The listing builds one solid part. Answer for the finished solid, in the listing's coordinates (mm). Round coordinates to 2 decimals unless told otherwise and drop trailing zeros. Write each loop counter-clockwise with the first axis right and the second up, starting at its lowest first coordinate (ties: lowest second). Pieces come first, ordered by that corner, then holes. Notation, with made-up numbers: M -26,-22 L -15,-22 A30 cw -15,16 Z; hole C -6.5,-30.75 d10. An arc over 180 degrees is marked long. Write each question's results on one line, items separated by ' | '.
Autodesk Inventor part; units mm, degrees
ref_plane "YZ Plane" through (0, 0, 0) normal (1, 0, 0) x (0, 1, 0)
ref_plane "XZ Plane" through (0, 0, 0) normal (0, 1, 0) x (-1, 0, 0)
ref_plane "XY Plane" through (0, 0, 0) normal (0, 0, 1) x (1, 0, 0)
sketch "スケッチ1" plane through (0, 0, 0) normal (0, 1, 0) x (-1, 0, 0)
  circle A0 centre (0, 0) radius 86.2565
  circle A1 centre (0, 0) radius 7.5
  dimension "d0" = 172.513
  dimension "d1" = 15
extrude "押し出し1" add sketch "スケッチ1" along normal blind 3
sketch "スケッチ2" plane through (0, 3, 0) normal (0, 1, 0) x (1, 0, 0)
  circle A0 centre (0, 0) radius 50.75
  point P0 (0, 50.75)
  point P1 (-50.75, 0)
  point P2 (0, -50.75)
  point P3 (50.75, 0)
  dimension "d4" = 101.5
  dimension "d7" = 360
hole "穴1" at (0, 3, -50.75) at (-50.75, 3, 0) at (0, 3, 50.75) at (50.75, 3, 0) direction (0, -1, 0) diameter 4.3 end through all
sketch "スケッチ3" plane through (0, 3, 0) normal (0, 1, 0) x (1, 0, 0)
  line L0 (0, 0) -> (86.2565, 0)
  circle A0 centre (0, 0) radius 86.2565
  circle A1 centre (0, 0) radius 7.5
  line L1 (0, 0) -> (60.9926, -60.9926)
  line L2 (-8.1772, -85.868) -> (-85.868, -8.1772)
  line L3 (85.868, 8.1772) -> (8.1772, 85.868)
  point P0 (8.1772, 85.868)
  point P1 (83.085, 0)
  point P2 (85.868, 8.1772)
  dimension "d16" = 45
  dimension "d64" = 66.5
extrude "押し出し2" cut sketch "スケッチ3" against normal blind 3 contours L3 A0 | A0 L2
sketch "スケッチ4" plane through (0, 3, 0) normal (0, 1, 0) x (1, 0, 0)
  circle A0 centre (0, 0) radius 7.5
  circle A1 centre (0, 0) radius 12
  line L0 (0, 0) -> (-8.4853, -8.4853)
  line L1 (0, 0) -> (-12, 0)
  point P0 (3.1058, -11.5911)
  point P1 (11.5911, -3.1058)
  point P2 (8.4853, 8.4853)
  point P3 (-3.1058, 11.5911)
  point P4 (-11.5911, 3.1058)
  dimension "d20" = 24
  dimension "d21" = 45
  dimension "d24" = 360
hole "穴2" at (-8.4853, 3, 8.4853) at (3.1058, 3, 11.5911) at (11.5911, 3, 3.1058) at (8.4853, 3, -8.4853) at (-3.1058, 3, -11.5911) at (-11.5911, 3, -3.1058) direction (0, -1, 0) diameter 4.3 end through all
sketch "スケッチ5" plane through (0, 3, 0) normal (0, 1, 0) x (1, 0, 0)
  arc A0 (-8.1772, -85.868) -> (85.868, 8.1772) centre (0, 0) ccw
  line L0 (5.2626, -86.0958) -> (-86.0958, 5.2626)
  arc A1 (8.1772, 85.868) -> (-85.868, -8.1772) centre (0, 0) ccw
  line L1 (-85.868, -8.1772) -> (-8.1772, -85.868)
  line L2 (-5.2626, 86.0958) -> (86.0958, -5.2626)
  line L3 (85.868, 8.1772) -> (8.1772, 85.868)
  line L4 (-85.868, -8.1772) -> (8.1772, 85.868)
  line L5 (-8.1772, -85.868) -> (85.868, 8.1772)
  line L6 (-73.6506, -7.1826) -> (7.1826, 73.6506)
  line L7 (80.2566, 13.7886) -> (-7.1826, -73.6506)
  line L8 (0, 0) -> (40.4166, 40.4166)
  circle A2 centre (0, 0) radius 74
  point P0 (-73.6506, -7.1826)
  point P1 (7.1826, 73.6506)
  point P2 (73.6506, 7.1826)
  dimension "d61" = 148
  dimension "d62" = 47
  dimension "d63" = 47
hole "穴3" at (-73.6506, 3, 7.1826) at (7.1826, 3, -73.6506) at (73.6506, 3, -7.1826) at (-7.1826, 3, 73.6506) direction (0, -1, 0) diameter 3.2 end through all
sketch "スケッチ6" plane through (0, 3, 0) normal (0, 1, 0) x (1, 0, 0)
  circle A0 centre (0, 0) radius 7.5
  circle A1 centre (0, 0) radius 70
  circle A2 centre (0, 0) radius 50
  circle A3 centre (7.1826, 73.6506) radius 1.6
  line L0 (0, 0) -> (7.1826, 73.6506)
  circle A4 centre (-73.6506, -7.1826) radius 1.6
  line L1 (0, 0) -> (-73.6506, -7.1826)
  line L2 (0, 0) -> (-11.469, 69.0541)
  line L3 (0, 0) -> (-69.0541, 11.469)
  circle A5 centre (0, 0) radius 25
  circle A6 centre (0, 50.75) radius 2.15
  line L4 (0, 0) -> (0, 50.75)
  line L5 (0, 0) -> (8.6824, 49.2404)
  line L6 (0, 0) -> (49.2404, 8.6824)
  circle A7 centre (50.75, 0) radius 2.15
  line L7 (0, 0) -> (50.75, 0)
  line L8 (0, 0) -> (-49.2404, -8.6824)
  line L9 (0, 0) -> (-8.6824, -49.2404)
  line L10 (0, 0) -> (11.469, -69.0541)
  line L11 (0, 0) -> (69.0541, -11.469)
  circle A8 centre (0, 0) radius 40
  point P0 (-4.3412, -24.6202)
  point P1 (-24.6202, -4.3412)
  point P2 (49.3243, -8.1921)
  point P3 (24.6622, -4.0961)
  point P4 (4.0961, -24.6622)
  point P5 (8.1921, -49.3243)
  point P6 (24.6202, 4.3412)
  point P7 (4.3412, 24.6202)
  point P8 (-24.6622, 4.0961)
  point P9 (-4.0961, 24.6622)
  point P10 (-8.1921, 49.3243)
  point P11 (-49.3243, 8.1921)
  point P12 (69.0541, -11.469)
  point P13 (11.469, -69.0541)
  point P14 (39.4595, -6.5537)
  point P15 (6.5537, -39.4595)
  point P16 (-39.4595, 6.5537)
  point P17 (-6.5537, 39.4595)
  dimension "d44" = 140
  dimension "d45" = 100
  dimension "d46" = 15
  dimension "d47" = 15
  dimension "d48" = 50
  dimension "d49" = 10
  dimension "d50" = 10
  dimension "d53" = 360
  dimension "d57" = 80
extrude "押し出し3" cut sketch "スケッチ6" against normal blind 10 contours A5 L5 A8 L6 | L11 A8 L10 A5 | A8 L5 A2 L6 | L11 A2 L10 A8 | A5 L3 A8 L2 | A5 L9 A8 L8 | L11 A1 L10 A2 | A8 L3 A2 L2 | A8 L9 A2 L8 | A2 L3 A1 L2
fillet "フィレット1" radius 5 14 edges at (-11.469, 1.5, -69.0541) (-69.0541, 1.5, -11.469) (-49.2404, 1.5, 8.6824) (-24.6202, 1.5, 4.3412) (-8.6824, 1.5, 49.2404) (-4.3412, 1.5, 24.6202) (11.469, 1.5, 69.0541) (69.0541, 1.5, 11.469) (24.6202, 1.5, -4.3412) (49.2404, 1.5, -8.6824) (8.6824, 1.5, -49.2404) (4.3412, 1.5, -24.6202) (-4.0961, 1.5, -24.6622) (-24.6622, 1.5, -4.0961)
equation "\"d64\" = Almiwidth4"
equation "\"d62\" = Almiwidth1"
equation "\"d63\" = Almiwidth1"
properties part number "baseplate_R2toR6" material "アルミニウム 6061"
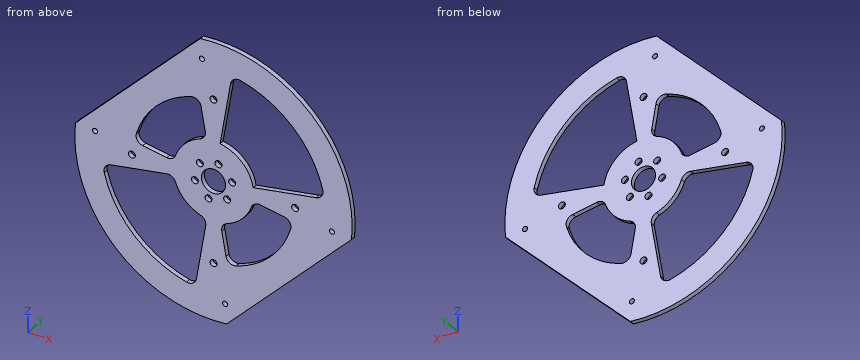
1) Section A-A (x = -37.5) is taken. Determine the outline of the cut face in (y, z), then the cut area to 3 significant figures.
Return value:
outline: M 0,-77.68 L 3,-77.68 L 3,-59.11 L 0,-59.11 Z; M 0,-6.23 L 3,-6.23 L 3,6.61 L 0,6.61 Z; M 0,33.07 L 3,33.07 L 3,56.55 L 0,56.55 Z | area: 165 mm²
2) Section B-B (z = 33.5) is taken. Determine the outline of the cut face in (x, y), then the cut area to 3 significant figures.
Return value:
outline: M -60.55,0 L -37.12,0 L -37.12,3 L -60.55,3 Z; M -5.91,0 L 5.56,0 L 5.56,3 L -5.91,3 Z; M 61.46,0 L 79.49,0 L 79.49,3 L 61.46,3 Z | area: 159 mm²
3) Find the intervals of material crossed by line 1 (Z direction, x = 0, y = 1.9); line 2 (X direction, y = 1.7, z = 15); line 3 (Z direction, x = -45, y = 2.4), in increasing order.
Return value:
line 1: -86.26 to -52.9, -48.6 to -7.5, 7.5 to 48.6, 52.9 to 86.26 | line 2: -79.05 to -47.7, -20 to 20, 68.08 to 84.94 | line 3: -73.59 to -53.62, -7.47 to 8.04, 21.79 to 49.05
4) Each of these flat-tipped pins is pushed along its axis until it touches: pin 1 (3.5 mm diameter, centred on x = 7.18, z = -73.65, fed in from +Y); pin 2 (1 mm diameter, centred on x = 53.5, y = 0.5, fed in from -Z); pin 3 (1 mm diameter, centred on y = 0.5, z = 67.5, fed in from -X). Where does it stop, or does it pass through?
Return value:
pin 1: y = 3 | pin 2: z = -41.05 | pin 3: x = -27.05
5) Section C-C (x = -56) is taken. Determine the outline of the cut face in (y, z), then the cut area to 3 significant figures.
Return value:
outline: M 0,-65.61 L 3,-65.61 L 3,-42 L 0,-42 Z; M 0,-9.3 L 3,-9.3 L 3,38.05 L 0,38.05 Z | area: 213 mm²
6) Section D-D (y = 2.2) is taken. State how many separate pieces and enclosed holes the cut face has, then the cut area to 3 significant figures.
Return value:
separate pieces: 1 | enclosed holes: 19 | area: 12,500 mm²
